Here's how the part is built. I have some questions about the finished solid (model axes, mm). Face numbers are marked on the shaded views. A direction names the side the tool comes from. Round coordinates to 2 decimals unless told otherwise and drop trailing zeros. Loops run counter-clockwise (first coordinate to the right, second up) from the corner with the lowest first, then second, coordinate; pieces in that order, holes last. Notation, with made-up numbers: (8, -7.75) -> (24, -7.75) arc R28 ccw to (24, 24.25) -> close; hole circle Ø9 at (66, 2). An arc over 180 degrees is marked (long way). Use one line per item in the form item = value. Start each with the question number.
Item 1: For the marked faces 1 and 2, which set-ups out of +Z, -Z, +X, -X, +Y, -Y let a thin tool reach every point of the face, with its end or its side?
Item 2: I'm going to push flat-ended pins straight in: pin 1 Ø6 at (x, z) = (2, 11.5) entering from +Y; pin 2 Ø6 at (x, z) = (6.5, 6) entering from -Y; pin 3 Ø6 at (y, z) = (9, 15) entering from +X; pin 4 Ø2 at (y, z) = (3, 11.5) entering from +X. Where does each tip first touch, or does it pass through?
Item 3: If we section it at A-A (x = 0): Write out the boundary of the cut face in (y, z) (3 decimals), then the cut area to 3 significant figures.
Item 4: Thinking about a two-plate mould opening in X: for the marked faces 3, 4 and 5, which applies, released by +X, released by -X, zero draft, split by the parting line, or undercut?
Item 5: If we section it at D-D (y = 6.5): Write out the boundary of the cut face in (x, z) (3 decimals), then the cut area to 3 significant figures.
Item 6: If I drill on L1, parallel to Z at x = 0, y = 3.25 (3 decimals); L2, parallel to Z at x = -2, y = 1.75; L3, parallel to Z at x = 0.25, y = 4.5, over which ranges is the centre line in solid material (lowest first)? Write a range as [from, to].
Item 7: If we section it at C-C (z = 2): Write out the boundary of the cut face in (x, y), then the cut area to 3 significant figures.
Item 8: If we section it at B-B (y = 8.75): Write out the boundary of the cut face in (x, z) (3 decimals).
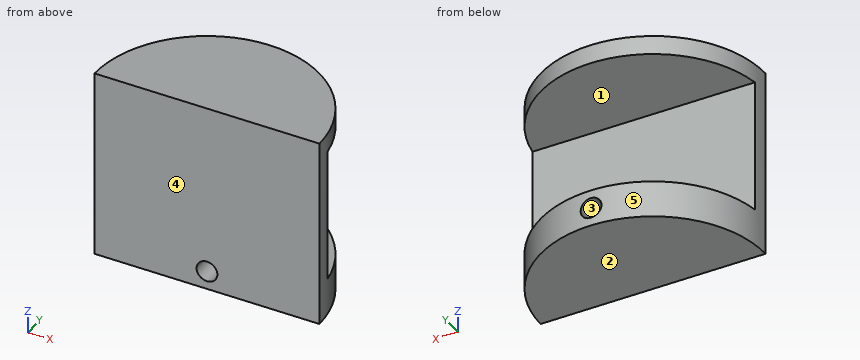
```python
from build123d import *

# Parameters (mm, degrees)
F1_DEPTH = 17
F3_W     = 22
F3_H     = 12
F4_DEPTH = 12
F5_R     = 0.925
F6_DEPTH = 12


with BuildPart() as f1:
    # F0 (on Top) → F1 (new body)
    with BuildSketch(Plane.XY):
        with BuildLine():
            Line((-10, 0), (10, 0))
            ThreePointArc((10, 0), (0, 10), (-10, 0))
        make_face()
    extrude(amount=F1_DEPTH)

    # F3 (on offset) → F4 (cut)
    with BuildSketch(Plane.XY.offset(3.3)):
        with Locations((-0.410548, 7.5)):
            Rectangle(F3_W, F3_H)
    extrude(amount=F4_DEPTH, mode=Mode.SUBTRACT)

    # F5 (on Front) → F6 (cut)
    with BuildSketch(Plane.XZ):
        with Locations((0, 1.65)):
            Circle(F5_R)
    extrude(amount=-F6_DEPTH, mode=Mode.SUBTRACT)


solid = f1.part
```
Values found:
q1.face_1 = +X, -X, +Y
q1.face_2 = -Z, +X, -X, +Y, -Y
q2.pin_1 = 1.5
q2.pin_2 = 0
q2.pin_3 = 7.99
q2.pin_4 = through
q3.outline = (0, 0) -> (10, 0) -> (10, 0.725) -> (0, 0.725) -> close; (0, 2.575) -> (10, 2.575) -> (10, 3.3) -> (1.5, 3.3) -> (1.5, 15.3) -> (10, 15.3) -> (10, 17) -> (0, 17) -> close
q3.area = 49.5 mm2
q4.face_3 = undercut
q4.face_4 = zero draft
q4.face_5 = split by the parting line
q5.outline = (-7.599, 0) -> (7.599, 0) -> (7.599, 3.3) -> (-7.599, 3.3) -> close; (-7.599, 15.3) -> (7.599, 15.3) -> (7.599, 17) -> (-7.599, 17) -> close; hole circle Ø1.85 at (0, 1.65)
q5.area = 73.3 mm2
q6.L1 = [0, 0.725], [2.575, 3.3], [15.3, 17]
q6.L2 = [0, 3.3], [15.3, 17]
q6.L3 = [0, 0.76], [2.54, 3.3], [15.3, 17]
q7.outline = (-10, 0) -> (-0.86, 0) -> (-0.86, 9.96) arc R10 ccw to start; (0.86, 0) -> (10, 0) arc R10 ccw to (0.86, 9.96) -> close
q7.area = 140 mm2
q8.outline = (-4.841, 0) -> (4.841, 0) -> (4.841, 3.3) -> (-4.841, 3.3) -> close; (-4.841, 15.3) -> (4.841, 15.3) -> (4.841, 17) -> (-4.841, 17) -> close; hole circle Ø1.85 at (0, 1.65)
